Build history of the part. All positions in model axes, mm. A direction names the side the tool comes from. Give positions to 0.01 mm unless a question says otherwise; leave off trailing zeros. Order: outer loops, then holes, each group sorted by start corner. A loop starts at its lowest first (then second) coordinate and runs counter-clockwise, first axis right, second up. Notation, with made-up numbers: (-27.75, 12) - (7.25, 12) arc R14 cw to (7.25, 24) - close; hole circle Ø8 at (-17, 63). An arc over 180 degrees is marked (long way). Answer in a Markdown table with one row per item.
```python
from build123d import *

# Parameters (mm, degrees)
F0_R     = 20
F1_DEPTH = 10
F2_DEPTH = 10


# Not quite as in the source:
# - a feature names something its author has since deleted; it is built from what else it names


with BuildPart() as f1:
    # F0 (on Top) → F1 (new body)
    with BuildSketch(Plane.XY):
        with Locations((31.903732568, 28.4272767603)):
            Circle(F0_R)
        Polygon((33.1302353929, 29.5670241683), (33.5040341896, 27.9349678601), (32.2775313647, 26.7952204522), (30.6772297431, 27.2875293524), (30.3034309464, 28.9195856605), (31.5299337713, 30.0593330685), align=None, mode=Mode.SUBTRACT)
    extrude(amount=F1_DEPTH)

    # F0 (on Top) → F2 (join)
    with BuildSketch(Plane.XY):
        with Locations((31.903732568, 28.4272767603)):
            Circle(F0_R)
        Polygon((33.1302353929, 29.5670241683), (33.5040341896, 27.9349678601), (32.2775313647, 26.7952204522), (30.6772297431, 27.2875293524), (30.3034309464, 28.9195856605), (31.5299337713, 30.0593330685), align=None, mode=Mode.SUBTRACT)
    extrude(amount=F2_DEPTH)


solid = f1.part
```
1. Drop flat-ended pins along their axis: P1, Ø5, axis at x = 18, z = 4, coming from the +Y side; P2, Ø1, axis at x = 46, z = 3, coming from the +Y side (3 decimals); P3, Ø3, axis at x = 30, z = 7, coming from the +Y side. Give the stop position or say it passes through.
Check result:
| item | result |
|---|---|
| P1 | stops at y = 44.86 |
| P2 | stops at y = 43.095 |
| P3 | stops at y = 48.42 |
2. Which spindle directions (+Z, -Z, +X, -X, +Y, -Y) get a long thin tool onto all of the face, cutting with end or side? Do faces 4 (the face through (31.489, 27.038, 4.93)), 5 (the face through (36, 29, 0)). Say none if no direction does.
Check result:
| item | result |
|---|---|
| face 4 | +Z, -Z |
| face 5 | -Z, +X, -X, +Y, -Y |
3. Cut at C-C on y = 18.5. Write the cut outline in (x, z).
Check result:
| item | result |
|---|---|
| outline | (14.54, 0) - (49.27, 0) - (49.27, 10) - (14.54, 10) - close |
4. Two-plate mould, pull along X, no slides. Class faces 1 (the face through (42.66, 45.29, 4.93)), 2 (the face through (30.493, 28.092, 4.93)), 3 (the face through (36, 29, 10)): +X half, -X half, draft (parallel to the pull), parting line (faces both ways), or undercut.
Check result:
| item | result |
|---|---|
| face 1 | parting line |
| face 2 | undercut |
| face 3 | draft |
5. Probe line 1 (Y direction, x = 32.5, z = 8.75); line 2 (Y direction, x = 15, z = 7.75); line 3 (Y direction, x = 22.5, z = 5.75). List the from-to ranges inside material, lowest first.
Check result:
| item | result |
|---|---|
| line 1 | y = 8.44 to 27, 29.76 to 48.42 |
| line 2 | y = 17.74 to 39.12 |
| line 3 | y = 10.78 to 46.08 |
6. Cut at B-B on x = 36.5. Write the cut outline in (y, z).
Check result:
| item | result |
|---|---|
| outline | (8.96, 0) - (47.89, 0) - (47.89, 10) - (8.96, 10) - close |
7. Cut at A-A on z = 1.75. Write the cut outline in (x, y), and give its area (3 significant figures).
Check result:
| item | result |
|---|---|
| outline | circle Ø40 at (31.9, 28.43); hole (30.3, 28.92) - (30.68, 27.29) - (32.28, 26.8) - (33.5, 27.93) - (33.13, 29.57) - (31.53, 30.06) - close |
| area | 1,250 mm² |
